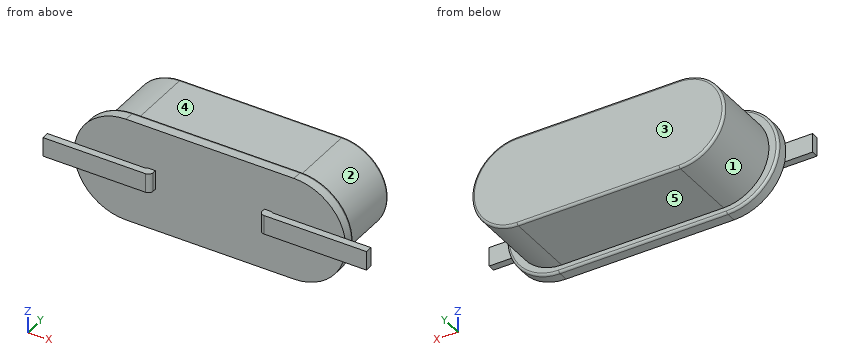
from build123d import *

# Parameters (mm, degrees)
BOSS_EXTRUDE1_DEPTH = 0.5
FILLET1_R           = 0.1
BOSS_EXTRUDE2_DEPTH = 3
FILLET2_R           = 0.1
SKETCH4_W           = 0.3
SKETCH4_H           = 0.8
BOSS_EXTRUDE3_DEPTH = 0.35
SKETCH5_W           = 0.8
SKETCH5_H           = 0.3
BOSS_EXTRUDE4_DEPTH = 4.2
FILLET3_R           = 0.2


with BuildPart() as part:
    # Sketch1 → Boss-Extrude1 (new body)
    with BuildSketch(Plane(origin=(0, 0, 0), x_dir=(1, 0, 0), z_dir=(0, 1, 0))):
        with BuildLine():
            Line((-3.525, 2.175), (3.525, 2.175))
            ThreePointArc((3.525, 2.175), (5.7, 0), (3.525, -2.175))
            Line((3.525, -2.175), (-3.525, -2.175))
            ThreePointArc((-3.525, -2.175), (-5.7, 0), (-3.525, 2.175))
        make_face()
    extrude(amount=BOSS_EXTRUDE1_DEPTH)

    # Fillet1
    fillet1_edges = [part.edges().sort_by_distance(p)[0] for p in [
        (5.7, 0.5, 0),
        (0, 0.5, -2.175),
        (-5.7, 0.5, 0),
        (0, 0.5, 2.175),
    ]]
    fillet(fillet1_edges, radius=FILLET1_R)

    # Sketch2 → Boss-Extrude2 (add)
    with BuildSketch(Plane(origin=(0, 0.5, 0), x_dir=(1, 0, 0), z_dir=(0, 1, 0))):
        with BuildLine():
            Line((-3.4, 1.9), (3.4, 1.9))
            ThreePointArc((3.4, 1.9), (5.3, 0), (3.4, -1.9))
            Line((3.4, -1.9), (-3.4, -1.9))
            ThreePointArc((-3.4, -1.9), (-5.3, 0), (-3.4, 1.9))
        make_face()
    extrude(amount=BOSS_EXTRUDE2_DEPTH)

    # Fillet2
    fillet2_edges = [part.edges().sort_by_distance(p)[0] for p in [
        (-5.3, 3.5, 0),
        (0, 3.5, 1.9),
        (5.3, 3.5, 0),
        (0, 3.5, -1.9),
    ]]
    fillet(fillet2_edges, radius=FILLET2_R)

    # Sketch4 → Boss-Extrude3 (add)
    with BuildSketch(Plane.XZ):
        with Locations((2.44, 0)):
            Rectangle(SKETCH4_W, SKETCH4_H)
        with Locations((-2.44, 0)):
            Rectangle(SKETCH4_W, SKETCH4_H)
    extrude(amount=BOSS_EXTRUDE3_DEPTH)

    # Sketch5 → Boss-Extrude4 (add)
    with BuildSketch(Plane.ZY.offset(2.59)):
        with Locations((0, -0.2)):
            Rectangle(SKETCH5_W, SKETCH5_H)
    boss_extrude4 = extrude(amount=BOSS_EXTRUDE4_DEPTH)

    # Mirror1: Boss-Extrude4 across plane
    add(boss_extrude4.mirror(Plane(origin=(0, 0, 0), x_dir=(0, 0, 1), z_dir=(1, 0, 0))))

    # Fillet3
    # the kernel refuses this fillet: 0.2 mm, written as the material it adds along each edge
    with BuildSketch(Plane(origin=(-2.59, -0.05, -0.4), x_dir=(-1, 0, 0), z_dir=(0, 0, 1))) as fillet3_piece_1:
        with BuildLine():
            CenterArc((0.132287566, -0.2), FILLET3_R, 90, 41.409622109)
            Line((0, -0.05), (0, 0))
            Line((0, 0), (0.132287566, 0))
        make_face()
    extrude(amount=0.8)
    with BuildSketch(Plane(origin=(2.59, -0.05, -0.4), x_dir=(0, 1, 0), z_dir=(0, 0, 1))) as fillet3_piece_2:
        with BuildLine():
            CenterArc((0.2, -0.132287566), FILLET3_R, 138.590377891, 41.409622109)
            Line((0, -0.132287566), (0, 0))
            Line((0, 0), (0.05, 0))
        make_face()
    extrude(amount=0.8)
    # the kernel refuses this fillet: 0.2 mm, written as the material it takes off along each edge
    with BuildSketch(Plane(origin=(2.29, -0.35, -0.9), x_dir=(0, 1, 0), z_dir=(0, 0, 1)), Plane(origin=(-2.29, -0.35, 0.9), x_dir=(0, 1, 0), z_dir=(0, 0, -1))) as fillet3_2_piece_1:
        with BuildLine():
            CenterArc((FILLET3_R, -FILLET3_R), FILLET3_R, 90, 90)
            Line((0, -FILLET3_R), (0, 0))
            Line((0, 0), (FILLET3_R, 0))
        make_face()
    extrude(amount=1.8, mode=Mode.SUBTRACT)


solid = part.part
Could you check a few things on this model? Use its own coordinates, in mm. Face numbers are marked on the shaded views. A direction names the side the tool comes from. Give positions to 0.01 mm unless a question says otherwise; leave off trailing zeros. Order: outer loops, then holes, each group sorted by start corner. A loop starts at its lowest first (then second) coordinate and runs counter-clockwise, first axis right, second up.
1. For pin 1 (1 mm diameter, centred on x = 5.5, y = 1.5, fed in from -Z); pin 2 (1.5 mm diameter, centred on x = -1.5, z = 0, fed in from -Y); pin 3 (1.5 mm diameter, centred on x = -4.5, y = 2, fed in from +Z), each with a flat end and sliding along its axis, tell me the tip position at first contact or that it passes through.
Answers below:
pin 1: stops at z = -1.02
pin 2: stops at y = 0
pin 3: stops at z = 1.87
2. I need wall thicknesses on L1, parallel to Z at x = 1.75, y = 3.35; L2, parallel to Y at x = 3.75, z = 1.4; L3, parallel to Z at x = -4, y = 0.65. Which ranges of each line are inside material? Lowest first, please.
Answers below:
L1: z = -1.9 to 1.9
L2: y = 0 to 3.5
L3: z = -1.8 to 1.8
3. Which directions (+Z, -Z, +X, -X, +Y, -Y) give clear straight access to the entire face, cutting with the end or side of a thin tool? Please do the marked faces 1, 2, 3, 4 and 5.
Answers below:
face 1: -X, +Y
face 2: +X, +Y
face 3: +Z, -Z, +X, -X, +Y
face 4: +Z, +X, -X, +Y
face 5: -Z, +X, -X, +Y
4. Suppose I cut it at A-A (z = 0). Write out the boundary of the cut face in (x, y), plus the area to 3 significant figures.
Answers below:
outline: (-6.79, -0.35) - (-2.49, -0.35) arc R0.2 ccw to (-2.29, -0.15) - (-2.29, 0) - (2.29, 0) - (2.29, -0.15) arc R0.2 ccw to (2.49, -0.35) - (6.79, -0.35) - (6.79, -0.05) - (2.72, -0.05) arc R0.2 cw to (2.59, 0) - (5.7, 0) - (5.7, 0.4) arc R0.1 ccw to (5.6, 0.5) - (5.3, 0.5) - (5.3, 3.4) arc R0.1 ccw to (5.2, 3.5) - (-5.2, 3.5) arc R0.1 ccw to (-5.3, 3.4) - (-5.3, 0.5) - (-5.6, 0.5) arc R0.1 ccw to (-5.7, 0.4) - (-5.7, 0) - (-2.59, 0) arc R0.2 cw to (-2.72, -0.05) - (-6.79, -0.05) - close
area: 40.2 mm2
5. Suppose I cut it at B-B (x = -0.5). Write out the boundary of the cut face in (y, z) (3 decimals), plus the area to 3 significant figures.
Answers below:
outline: (0, -2.175) - (0.4, -2.175) arc R0.1 ccw to (0.5, -2.075) - (0.5, -1.9) - (3.4, -1.9) arc R0.1 ccw to (3.5, -1.8) - (3.5, 1.8) arc R0.1 ccw to (3.4, 1.9) - (0.5, 1.9) - (0.5, 2.075) arc R0.1 ccw to (0.4, 2.175) - (0, 2.175) - close
area: 13.6 mm2
6. Suppose I cut it at C-C (y = 2.05). Write out the boundary of the cut face in (x, z), plus the area to 3 significant figures.
Answers below:
outline: (-3.4, -1.9) - (3.4, -1.9) arc R1.9 ccw to (3.4, 1.9) - (-3.4, 1.9) arc R1.9 ccw to start
area: 37.2 mm2
